Geometry check sheet. Reference: drawing and pictorial views, mm from the part's lowest x, y, z. Give positions to 0.01 mm unless a question says otherwise; leave off trailing zeros. Write each loop counter-clockwise with the first axis right and the second up, starting at its lowest first coordinate (ties: lowest second). Pieces come first, ordered by that corner, then holes. Notation, with made-up numbers: M 32.5,50 L 55.5,50 A8 cw 55.5,54 Z; hole C 53,-40 d7. An arc over 180 degrees is marked long. Answer as a JSON object with one key per item and string values.
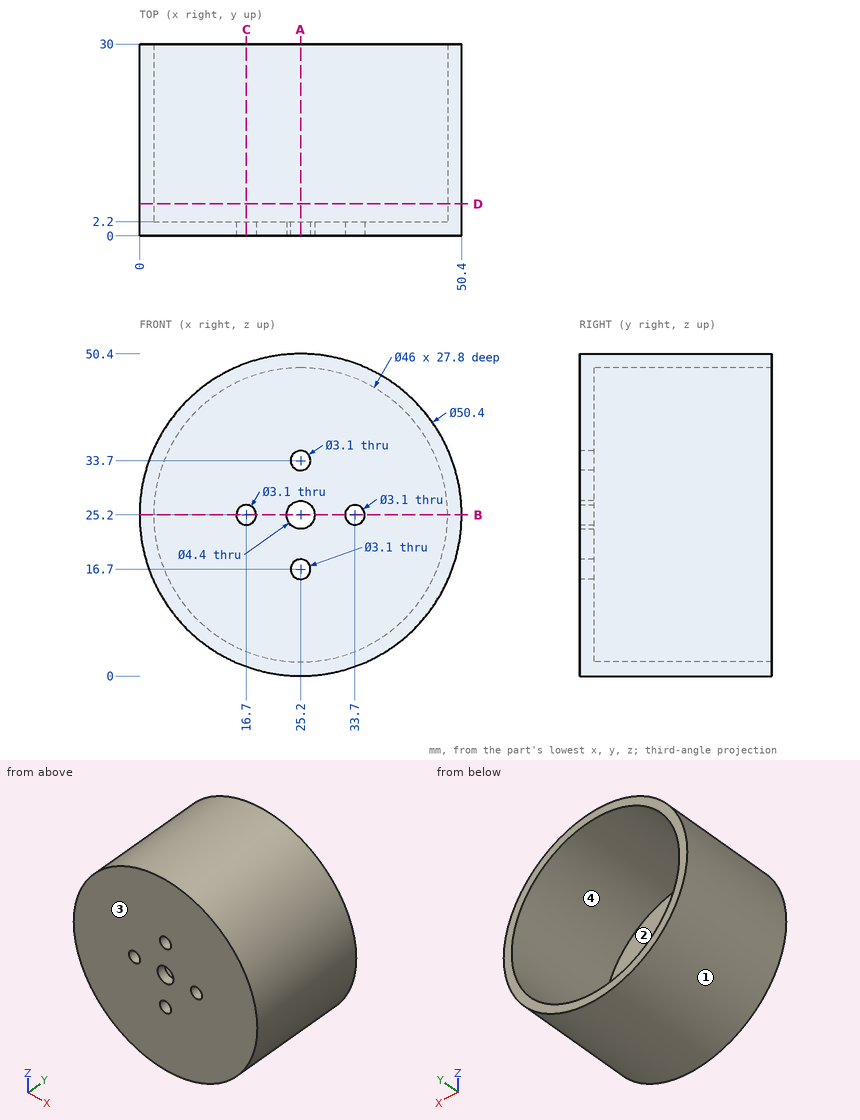
1) Go/stop test with flat-tipped pins: pin 1 (23 mm diameter, centred on x = 30.5, z = 27, fed in from +Y); pin 2 (1.9 mm diameter, centred on x = 25.2, z = 16.7, fed in from +Y); pin 3 (12 mm diameter, centred on y = 11, z = 44, fed in from -X); pin 4 (6 mm diameter, centred on y = 25.5, z = 14, fed in from +X). Record where each tip stops, or that it passes through.
Completed:
{"pin 1": "stops at y = 2.2", "pin 2": "passes through", "pin 3": "stops at x = 3.49", "pin 4": "stops at x = 49.03"}
2) Section check B-B on z = 25.2. Record the boundary of the cut face in (x, y).
Completed:
{"outline": "M 0,0 L 15.15,0 L 15.15,2.2 L 2.2,2.2 L 2.2,30 L 0,30 Z; M 18.25,0 L 23,0 L 23,2.2 L 18.25,2.2 Z; M 27.4,0 L 32.15,0 L 32.15,2.2 L 27.4,2.2 Z; M 35.25,0 L 50.4,0 L 50.4,30 L 48.2,30 L 48.2,2.2 L 35.25,2.2 Z"}
3) Section check C-C on x = 16.7. Record the boundary of the cut face in (y, z).
Completed:
{"outline": "M 0,1.48 L 30,1.48 L 30,3.83 L 2.2,3.83 L 2.2,23.65 L 0,23.65 Z; M 0,26.75 L 2.2,26.75 L 2.2,46.57 L 30,46.57 L 30,48.92 L 0,48.92 Z"}
4) Thickness scan on L1, parallel to X at y = 1, z = 25.2; L2, parallel to X at y = 19.75, z = 25.2; L3, parallel to Z at x = 44.5, y = 6. Record the ranges inside material, lowest first.
Completed:
{"L1": "x = 0 to 15.15, 18.25 to 23, 27.4 to 32.15, 35.25 to 50.4", "L2": "x = 0 to 2.2, 48.2 to 50.4", "L3": "z = 9 to 12.69, 37.71 to 41.4"}
5) Release check for a two-part mould opening along X. For the marked faces 1, 2, 3 and 4 record: pulls with the +X half, pulls with the -X half, needs draft (parallel to the pull), parting line crosses it, or undercut.
Completed:
{"face 1": "parting line crosses it", "face 2": "undercut", "face 3": "needs draft", "face 4": "undercut"}
6) Section check A-A on x = 25.2. Record the boundary of the cut face in (y, z), and give its area (3 significant figures).
Completed:
{"outline": "M 0,0 L 30,0 L 30,2.2 L 2.2,2.2 L 2.2,15.15 L 0,15.15 Z; M 0,18.25 L 2.2,18.25 L 2.2,23 L 0,23 Z; M 0,27.4 L 2.2,27.4 L 2.2,32.15 L 0,32.15 Z; M 0,35.25 L 2.2,35.25 L 2.2,48.2 L 30,48.2 L 30,50.4 L 0,50.4 Z", "area": "210 mm2"}
7) Section check D-D on y = 5. Record the boundary of the cut face in (x, z).
Completed:
{"outline": "C 25.2,25.2 d50.4; hole C 25.2,25.2 d46"}
